Source: CAD feature listing. Evaluate the final solid. Frame: model axes, mm. A direction names the side the tool comes from. Give positions to 0.01 mm unless a question says otherwise; leave off trailing zeros. Order: outer loops, then holes, each group sorted by start corner. A loop starts at its lowest first (then second) coordinate and runs counter-clockwise, first axis right, second up.
from build123d import *

# Parameters (mm, degrees)
SKETCH_1_R                      = 19
SKETCH_1_R_2                    = 13.5
EXTRUDE_1_DEPTH                 = 1.5
SKETCH_2_W                      = 5
SKETCH_2_H                      = 5
EXTRUDE_2_DEPTH                 = 1.5
PATTERN_CIRCULAR_2_COUNT        = 12
SKETCH_6_R                      = 1.75
CUT_EXTRUDE_1_DEPTH             = 0.1
PATTERN_CIRCULAR_3_COUNT        = 12
SKETCH_7_R                      = 1
CUT_EXTRUDE_2_DEPTH             = 28.037011669
EXTRUDE_3_DEPTH                 = 0.7
PATTERN_CIRCULAR_4_COUNT        = 5
PATTERN_CIRCULAR_4_ANGLE        = 120
PATTERN_CIRCULAR_5_COUNT        = 2
PATTERN_CIRCULAR_5_ANGLE        = 60
PATTERN_CIRCULAR_6_COUNT        = 5
PATTERN_CIRCULAR_6_ANGLE        = 120
PATTERN_CIRCULAR_6_COPY_1_DEPTH = 0.7
PATTERN_CIRCULAR_6_COPY_2_DEPTH = 0.7
PATTERN_CIRCULAR_6_COPY_3_DEPTH = 0.7


with BuildPart() as part:
    # ｽｹｯﾁ1 → ﾎﾞｽ - 押し出し1 (new body)
    with BuildSketch(Plane.XY):
        Circle(SKETCH_1_R)
        Circle(SKETCH_1_R_2, mode=Mode.SUBTRACT)
    extrude(amount=EXTRUDE_1_DEPTH)

    # ｽｹｯﾁ2 → ﾎﾞｽ - 押し出し2 (add)
    with BuildSketch(Plane.XY.offset(1.5)):
        with Locations((0, 16.1)):
            Rectangle(SKETCH_2_W, SKETCH_2_H)
    extrude_2 = extrude(amount=EXTRUDE_2_DEPTH)

    # 円形ﾊﾟﾀｰﾝ2: ﾎﾞｽ - 押し出し2 ×12 about axis
    pattern_circular_2_axis = Axis((0, 0, 0), (0, 0, 1))
    for i in range(1, PATTERN_CIRCULAR_2_COUNT):
        add(extrude_2.rotate(pattern_circular_2_axis, i * 360 / PATTERN_CIRCULAR_2_COUNT))

    # ｽｹｯﾁ6 → ｶｯﾄ - 押し出し1 (cut)
    with BuildSketch(Plane.XY.offset(3)):
        with Locations((0, 16.1)):
            Circle(SKETCH_6_R)
        Polygon((-2.5, 18.1), (-2, 18.6), (-2.5, 18.6), align=None)
    cut_extrude_1 = extrude(amount=-CUT_EXTRUDE_1_DEPTH, mode=Mode.SUBTRACT)

    # 円形ﾊﾟﾀｰﾝ3: ｶｯﾄ - 押し出し1 ×12 about axis
    pattern_circular_3_axis = Axis((0, 0, 0), (0, 0, 1))
    for i in range(1, PATTERN_CIRCULAR_3_COUNT):
        add(cut_extrude_1.rotate(pattern_circular_3_axis, i * 360 / PATTERN_CIRCULAR_3_COUNT), mode=Mode.SUBTRACT)

    # ｽｹｯﾁ7 → ｶｯﾄ - 押し出し2 (cut, through all)
    with BuildSketch(Plane(origin=(0, 0, 0), x_dir=(-1, 0, 0), z_dir=(0, 0, -1))):
        with Locations((4.464628528, -16.662220503)):
            Circle(SKETCH_7_R)
        with Locations((-4.464628528, 16.662220503)):
            Circle(SKETCH_7_R)
    extrude(amount=-CUT_EXTRUDE_2_DEPTH, mode=Mode.SUBTRACT)

    # ｽｹｯﾁ8 → ﾎﾞｽ - 押し出し3 (add)
    with BuildSketch(Plane.XY.offset(1.5)):
        Polygon((4.527475052, -15.351285603), (3.754734391, -15.558340839), (4.190189437, -17.183481193), (4.962930098, -16.976425957), align=None)
    extrude_3 = extrude(amount=EXTRUDE_3_DEPTH)

    # 円形ﾊﾟﾀｰﾝ4: ﾎﾞｽ - 押し出し3 ×5 about axis
    pattern_circular_4_axis = Axis((0, 0, 0), (0, 0, 1))
    for i in range(1, PATTERN_CIRCULAR_4_COUNT):
        add(extrude_3.rotate(pattern_circular_4_axis, i * PATTERN_CIRCULAR_4_ANGLE / (PATTERN_CIRCULAR_4_COUNT - 1)))

    # 円形ﾊﾟﾀｰﾝ5: ﾎﾞｽ - 押し出し3 ×2 about axis
    pattern_circular_5_axis = Axis((0, 0, 0), (0, 0, -1))
    for i in range(1, PATTERN_CIRCULAR_5_COUNT):
        add(extrude_3.rotate(pattern_circular_5_axis, i * PATTERN_CIRCULAR_5_ANGLE / (PATTERN_CIRCULAR_5_COUNT - 1)))

    # 円形ﾊﾟﾀｰﾝ6: ﾎﾞｽ - 押し出し3 ×5 about axis, 1 skipped
    pattern_circular_6_axis = Axis((0, 0, 1.5), (0, 0, -1))
    add([extrude_3.rotate(pattern_circular_6_axis, i * PATTERN_CIRCULAR_6_ANGLE / (PATTERN_CIRCULAR_6_COUNT - 1)) for i in range(1, PATTERN_CIRCULAR_6_COUNT) if i not in (1,)])

    # 円形ﾊﾟﾀｰﾝ6 copy 1 sketch → 円形ﾊﾟﾀｰﾝ6 copy 1 (add)
    with BuildSketch(Plane(origin=(0, 0, 1.5), x_dir=(-0.5000000000000044, -0.866025403784436, 0), z_dir=(0, 0, 1))):
        Polygon((4.527475052, -15.351285603), (3.754734391, -15.558340839), (4.190189437, -17.183481193), (4.962930098, -16.976425957), align=None)
    extrude(amount=PATTERN_CIRCULAR_6_COPY_1_DEPTH)

    # 円形ﾊﾟﾀｰﾝ6 copy 2 sketch → 円形ﾊﾟﾀｰﾝ6 copy 2 (add)
    with BuildSketch(Plane(origin=(0, 0, 1.5), x_dir=(-0.8660254037844418, -0.49999999999999456, 0), z_dir=(0, 0, 1))):
        Polygon((4.527475052, -15.351285603), (3.754734391, -15.558340839), (4.190189437, -17.183481193), (4.962930098, -16.976425957), align=None)
    extrude(amount=PATTERN_CIRCULAR_6_COPY_2_DEPTH)

    # 円形ﾊﾟﾀｰﾝ6 copy 3 sketch → 円形ﾊﾟﾀｰﾝ6 copy 3 (add)
    with BuildSketch(Plane(origin=(0, 0, 1.5), x_dir=(-1, 0, 0), z_dir=(0, 0, 1))):
        Polygon((4.527475052, -15.351285603), (3.754734391, -15.558340839), (4.190189437, -17.183481193), (4.962930098, -16.976425957), align=None)
    extrude(amount=PATTERN_CIRCULAR_6_COPY_3_DEPTH)


solid = part.part
(1) Access query for faces 1 (the flat face through (12, -12, 2.2)), 2 (the flat face through (-16.3, 4.4, 2.2)). Directions: +Z, -Z, +X, -X, +Y, -Y. A direction counts if a zero-diameter tool reaches every point of the face in a straight line with its end or side. Return the directions, or none.
(2) Section A-A, the plane y = 0. Return loops of the section in (x, z), plus the area to 3 significant figures.
(3) Pin query (flat end, axial travel): pin 1 Ø1.8 at (x, y) = (-14, 8.5) entering from +Z; pin 2 Ø1 at (y, z) = (-13.5, 1) entering from +X; pin 3 Ø1.5 at (y, z) = (-10.5, 1) entering from +X. Return the tip coordinate at first contact, or that it passes through.
(4) Line query: line 1 along X through (y, z) = (0, 2.7); line 2 along X through (y, z) = (-0.5, 0.35); line 3 along X through (y, z) = (14.5, 1.6). Output: solid intervals per line, ascending.
(5) Draft query along Y for faces 3 (the flat face through (-11.795, 6.77, 2.24)), 4 (the flat face through (-2, 17, 3)). Return one class per face: +Y half, -Y half, draft (parallel to the pull), parting line (faces both ways), or undercut.
Checks:
1. face 1: +Z
1. face 2: +Z, -X
2. outline: (-19, 0) - (-13.5, 0) - (-13.5, 1.5) - (-13.6, 1.5) - (-13.6, 3) - (-14.35, 3) - (-14.35, 2.9) - (-17.85, 2.9) - (-17.85, 3) - (-18.6, 3) - (-18.6, 1.5) - (-19, 1.5) - close; (13.5, 0) - (19, 0) - (19, 1.5) - (18.6, 1.5) - (18.6, 3) - (17.85, 3) - (17.85, 2.9) - (14.35, 2.9) - (14.35, 3) - (13.6, 3) - (13.6, 1.5) - (13.5, 1.5) - close
2. area: 30.8 mm2
3. pin 1: stops at z = 2.9
3. pin 2: stops at x = 13.86
3. pin 3: stops at x = 16.31
4. line 1: x = -18.6 to -13.6, 13.6 to 18.6
4. line 2: x = -18.99 to -13.49, 13.49 to 18.99
4. line 3: x = -11.26 to -5.48, -2.5 to 2.5, 5.48 to 11.26
5. face 3: undercut
5. face 4: draft
